Check sheet for the modelled part. Datum: model origin and axes. Units: mm. A direction names the side the tool comes from. Coordinates: 2 decimals unless noted, no trailing zeros. Write each loop counter-clockwise with the first axis right and the second up, starting at its lowest first coordinate (ties: lowest second). Pieces come first, ordered by that corner, then holes. Notation, with made-up numbers: (81, 52.25) - (95, 52.25) arc R19 cw to (95, 79.25) - close; hole circle Ø5 at (-2.5, -31.75). An arc over 180 degrees is marked (long way). Use one line per item in the form item = value. Start each with the question number.
1. Scan lines: line 1 along X through (y, z) = (-19.05, 11) (3 decimals); line 2 along Y through (x, z) = (-6.25, 11); line 3 along Y through (x, z) = (0, 10) (3 decimals). Record each from-to range of solid material in increasing order.
2. Cross-section at D-D on x = 0. Record the boundary of the cut face in (y, z) (3 decimals).
3. Draft check along Y on faces 1 (the face through (8.77, -10.45, 12.52)), 2 (the face through (-8.305, -14.226, 12.522)), 3 (the face through (-14.605, -9, 13)). Enter one of: +Y half, -Y half, draft (parallel to the pull), parting line (faces both ways), or undercut.
4. Go/stop test with flat-tipped pins: pin 1 Ø4 at (x, z) = (2.5, 3) entering from -Y; pin 2 Ø8 at (y, z) = (-8.5, 16) entering from +X; pin 3 Ø2 at (x, z) = (7, 16.5) entering from +Y; pin 4 Ø7 at (x, y) = (-8.89, -19.05) entering from +Z. Record where each tip stops, or that it passes through.
5. Cross-section at B-B on y = -5.5. Record the boundary of the cut face in (x, z) (3 decimals), then the cut area to 3 significant figures.
6. Cross-section at C-C on z = 10.25. Record the boundary of the cut face in (x, y) (3 decimals), then the cut area to 3 significant figures.
7. Tool access check on faces 4 (the face through (-12.7, -10, 13)), 5 (the face through (-13, -4, 25.4)). Record the directions out of +Z, -Z, +X, -X, +Y, -Y that give a thin tool (end or side, any length) a straight path to the whole face; none if there is none.
8. Cross-section at A-A on x = -11.5. Record the boundary of the cut face in (y, z), then the cut area to 3 significant figures.
```python
from build123d import *

# Parameters (mm, degrees)
F1_DEPTH = 25.4
F2_R     = 0.254


with BuildPart() as f1:
    # F0 (on Top) → F1 (new body)
    with BuildSketch(Plane.XY):
        with BuildLine():
            Line((-12.7, -19.05), (-12.7, 0))
            ThreePointArc((-12.7, 0), (5.367252, 11.510109), (8.163403, -9.728764))
            Line((8.163403, -9.728764), (9.387913, -11.188079))
            ThreePointArc((9.387913, -11.188079), (6.17234, 13.236625), (-14.605, 0))
            Line((-14.605, 0), (-14.605, -19.05))
            ThreePointArc((-14.605, -19.05), (-5.23671, -23.444849), (-7.845702, -13.431222))
            Line((-7.845702, -13.431222), (-8.89, -15.24))
            ThreePointArc((-8.89, -15.24), (-6.195923, -21.744077), (-12.7, -19.05))
        make_face()
    extrude(amount=F1_DEPTH)

    # F2
    f2_edges = [f1.edges().sort_by_distance(p)[0] for p in [
        (8.163403, -9.728764, 12.7),
        (9.387913, -11.188079, 12.7),
        (-7.845702, -13.431222, 12.7),
        (-8.89, -15.24, 12.7),
    ]]
    fillet(f2_edges, radius=F2_R)


solid = f1.part
```
Final values:
q1.line_1 = -14.605 to -12.7, -5.08 to -3.175
q1.line_2 = -24.12 to -21.8, -16.3 to -13.98, 11.06 to 13.2
q1.line_3 = 12.7 to 14.605
q2.outline = (12.7, 0) - (14.605, 0) - (14.605, 25.4) - (12.7, 25.4) - close
q3.face_1 = -Y half
q3.face_2 = undercut
q3.face_3 = draft
q4.pin_1 = 11.88
q4.pin_2 = 13.89
q4.pin_3 = 13.32
q4.pin_4 = through
q5.outline = (-14.605, 0) - (-12.7, 0) - (-12.7, 25.4) - (-14.605, 25.4) - close; (11.447, 0) - (13.53, 0) - (13.53, 25.4) - (11.447, 25.4) - close
q5.area = 101 mm²
q6.outline = (-14.605, -19.05) arc R5.715 ccw (long way) to (-7.663, -13.468) arc R0.254 ccw to (-7.937, -13.589) - (-8.683, -14.881) arc R0.254 ccw to (-8.49, -15.261) arc R3.81 cw (long way) to (-12.7, -19.05) - (-12.7, 0) arc R12.7 cw (long way) to (8.353, -9.567) arc R0.254 ccw to (8.325, -9.921) - (9.223, -10.992) arc R0.254 ccw to (9.584, -11.02) arc R14.605 ccw (long way) to (-14.605, 0) - close
q6.area = 182 mm²
q7.face_4 = +Z, -Z
q7.face_5 = +Z, +X, -X, +Y, -Y
q8.outline = (-24.13, 0) - (-21.83, 0) - (-21.83, 25.4) - (-24.13, 25.4) - close; (5.39, 0) - (9, 0) - (9, 25.4) - (5.39, 25.4) - close
q8.area = 150 mm²
